Can you work these out from the model? Positions are in its coordinate system, mm. A direction names the side the tool comes from. Coordinates: 2 decimals unless noted, no trailing zeros. Write each loop counter-clockwise with the first axis right and the second up, starting at its lowest first coordinate (ties: lowest second). Pieces come first, ordered by that corner, then holes. Notation, with made-up numbers: (-6.5, -0.5) - (-1.5, -0.5) arc R18 ccw to (-1.5, 4.5) - close; hole circle Ø2 at (32.25, -27.5). An arc over 180 degrees is marked (long way). Write each question's results on one line, items separated by ' | '. Start each with the question number.
Autodesk Inventor part; units mm, degrees
ref_plane "YZ Plane" through (0, 0, 0) normal (1, 0, 0) x (0, 1, 0)
ref_plane "XZ Plane" through (0, 0, 0) normal (0, 1, 0) x (-1, 0, 0)
ref_plane "XY Plane" through (0, 0, 0) normal (0, 0, 1) x (1, 0, 0)
sketch "Sketch1" plane through (0, 0, 0) normal (1, 0, 0) x (0, 1, 0)
  circle A0 centre (0, 0) radius 6.096
  arc A1 (0, 9.906) -> (0, -9.906) centre (0, 0) ccw
  line L0 (0, 9.906) -> (12.7, 9.906)
  line L1 (12.7, 9.906) -> (12.7, -9.906)
  line L2 (12.7, -9.906) -> (0, -9.906)
  arc A2 (0, -9.906) -> (0, 9.906) centre (0, 0) ccw construction
  dimension "d0" = 12.192
  dimension "d1" = 3.81
  dimension "d2" = 12.7
extrude "Extrusion1" add sketch "Sketch1" along normal blind 3.175
sketch "Sketch3" plane through (0, 12.7, 9.906) normal (0, 1, 0) x (1, 0, 0)
  line L0 (-12.065, 41.656) -> (3.175, 41.656)
  line L1 (3.175, 41.656) -> (3.175, -21.844)
  line L2 (3.175, -21.844) -> (-12.065, -21.844)
  line L3 (-12.065, -21.844) -> (-12.065, 41.656)
  line L4 (3.175, 19.812) -> (3.175, 0)
  circle A0 centre (-4.445, 33.782) radius 2.5527
  circle A1 centre (-4.445, -13.97) radius 2.5527
  line L5 (-12.065, 9.906) -> (3.175, 9.906) construction
  point P0 (0, 9.906)
  dimension "d6" = 63.5
  dimension "d7" = 15.24
  dimension "d8" = 5.1054
  dimension "d9" = 47.752
  dimension "d10" = 7.62
extrude "Extrusion2" add sketch "Sketch3" along normal blind 2.54
fillet "Fillet1" radius 8.255 2 edges at (1.5875, 12.7, -9.906) (1.5875, 12.7, 9.906)
fillet "Fillet2" radius 1.27 1 edges at (0, 12.7, 0)
fillet "Fillet3" radius 3.175 4 edges at (-12.065, 13.97, -31.75) (3.175, 13.97, -31.75) (3.175, 13.97, 31.75) (-12.065, 13.97, 31.75)
properties part number "ToggleSwitchBracket"
Q1. For faces 4 (the face through (0, 5.4, 3.3)), 5 (the face through (2, 2, 9.906)), 6 (the face through (2, 2, -9.906)), which set-ups out of +Z, -Z, +X, -X, +Y, -Y let a thin tool reach every point of the face, with its end or its side?
Q2. I need wall thicknesses on line 1 along Z through (x, y) = (1.8, 0); line 2 along Y through (x, z) = (-3.75, -2.5); line 3 along X through (y, z) = (-7.5, -3) (3 decimals). Which ranges of each line are inside material? Lowest first, please. Write a range as from..to.
Q3. Thinking about a two-plate mould opening in Z: for faces 1 (the face through (-4, 14, 31.75)), 2 (the face through (2.27, 13.988, -30.795)), 3 (the face through (-6.47, 13.95, 22.32)), which applies, pulls with the +Z half, pulls with the -Z half, needs draft (parallel to the pull), parting line crosses it, or undercut?
Q4. If we section it at A-A (z = 0): Please give me the cut outline in (x, y) (3 decimals), then the cut area to 3 significant figures.
Q5. If we section it at B-B (y = 3.5): Please give me the cut outline in (x, z) (3 decimals).
Q6. I'm going to push flat-ended pins straight in: pin 1 Ø6.5 at (x, z) = (-4.445, -23.876) entering from -Y; pin 2 Ø3.5 at (x, y) = (1.5, 2.5) entering from +Z; pin 3 Ø10.5 at (y, z) = (5, -6) entering from -X. Where does each tip first touch, or does it pass through?
Q7. If we section it at D-D (x = -3): Please give me the cut outline in (y, z), then the cut area to 3 significant figures.
Q8. If we section it at C-C (x = 1.25): Please give me the cut outline in (y, z) (3 decimals).
Answer list:
1) face 4: +Z, -Z, -X, -Y | face 5: +Z, +X, -X, -Y | face 6: -Z, +X, -X, -Y
2) line 1: z = -9.91..-6.1, 6.1..9.91 | line 2: y = 12.7..15.24 | line 3: x = 0..3.175
3) face 1: pulls with the +Z half | face 2: pulls with the -Z half | face 3: undercut
4) outline: (-12.065, 12.7) - (-1.27, 12.7) arc R1.27 cw to (0, 11.43) - (0, 6.096) - (3.175, 6.096) - (3.175, 15.24) - (-12.065, 15.24) - close; (0, -9.906) - (3.175, -9.906) - (3.175, -6.096) - (0, -6.096) - close | area: 72.1 mm2
5) outline: (0, -9.906) - (3.175, -9.906) - (3.175, -4.991) - (0, -4.991) - close; (0, 4.991) - (3.175, 4.991) - (3.175, 9.906) - (0, 9.906) - close
6) pin 1: stops at y = 12.7 | pin 2: stops at z = 9.91 | pin 3: stops at x = 0
7) outline: (12.7, -31.75) - (15.24, -31.75) - (15.24, -25.98) - (12.7, -25.98) - close; (12.7, -21.77) - (15.24, -21.77) - (15.24, 21.77) - (12.7, 21.77) - close; (12.7, 25.98) - (15.24, 25.98) - (15.24, 31.75) - (12.7, 31.75) - close | area: 140 mm2
8) outline: (0, -9.906) - (4.445, -9.906) arc R8.255 cw to (12.7, -18.161) - (12.7, -31.494) - (15.24, -31.494) - (15.24, 31.494) - (12.7, 31.494) - (12.7, 18.161) arc R8.255 cw to (4.445, 9.906) - (0, 9.906) arc R9.906 ccw to start; hole circle Ø12.192 at (0, 0)
